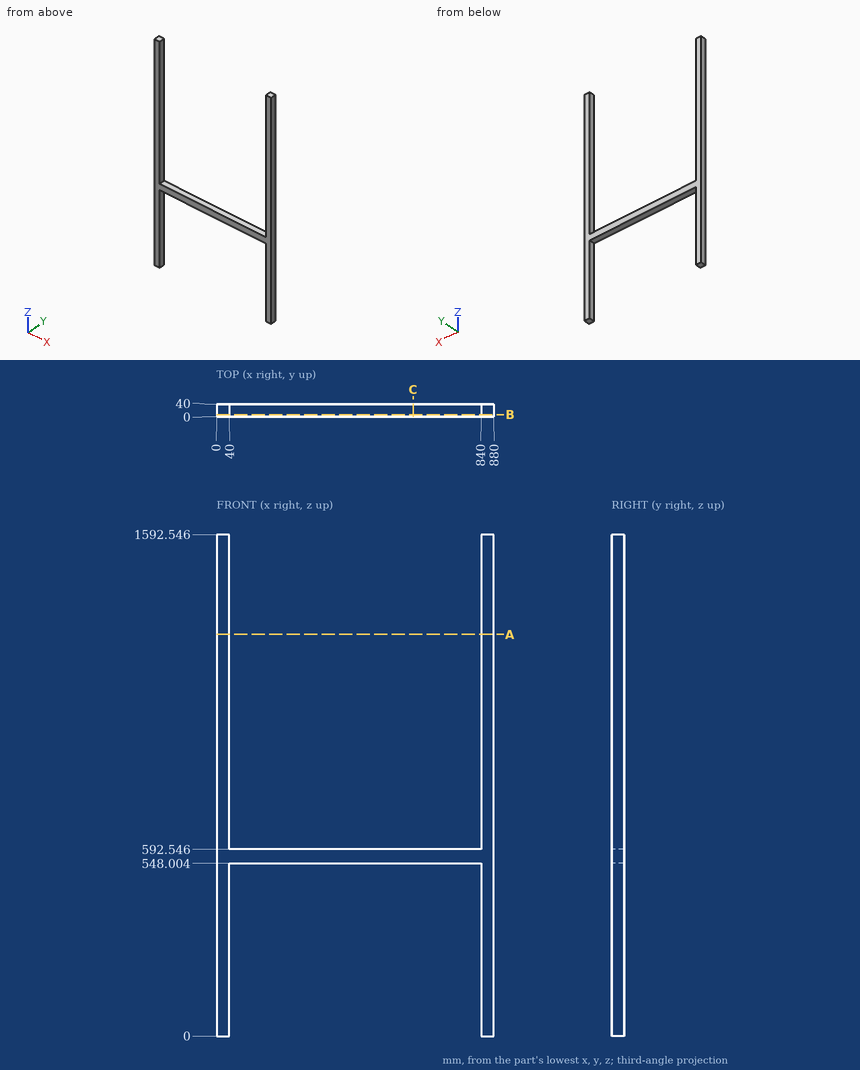
Could you check a few things on this drawing? It's one solid part, dimensions in mm from its lowest x, y, z. Give positions to 0.01 mm unless a question says otherwise; leave off trailing zeros. Write each loop counter-clockwise with the first axis right and the second up, starting at its lowest first coordinate (ties: lowest second). Pieces come first, ordered by that corner, then holes. Notation, with made-up numbers: (5.25, 29.25) -> (55.25, 29.25) arc R33 ccw to (55.25, 65.25) -> close; hole circle Ø6 at (-27.75, 86.25). An arc over 180 degrees is marked (long way). Answer as a JSON object with one key per item and string values.
Q1. Please list where these lines run through material, in increasing order: L1, parallel to X at y = 7.5, z = 769; L2, parallel to Z at x = 351.5, y = 35.
Taken from the geometry:
{"L1": "x = 0 to 40, 840 to 880", "L2": "z = 548 to 592.55"}
Q2. Suppose I cut it at C-C on x = 624. Write out the boundary of the cut face in (y, z).
Taken from the geometry:
{"outline": "(0, 548) -> (40, 548) -> (40, 592.55) -> (0, 592.55) -> close"}
Q3. Suppose I cut it at B-B on y = 6. Write out the boundary of the cut face in (x, z).
Taken from the geometry:
{"outline": "(0, 0) -> (40, 0) -> (40, 548) -> (840, 548) -> (840, 0) -> (880, 0) -> (880, 1592.55) -> (840, 1592.55) -> (840, 592.55) -> (40, 592.55) -> (40, 1592.55) -> (0, 1592.55) -> close"}
Q4. Will these pins go through, and if not, where does the flat tip stop? pin 1 Ø4 at (x, y) = (251.5, 29.5) entering from -Z; pin 2 Ø1 at (x, y) = (167, 4) entering from +Z; pin 3 Ø12 at (x, z) = (745.5, 600) entering from +Y.
Taken from the geometry:
{"pin 1": "stops at z = 548", "pin 2": "stops at z = 592.55", "pin 3": "passes through"}
Q5. Suppose I cut it at A-A on z = 1275.5. Write out the boundary of the cut face in (x, y).
Taken from the geometry:
{"outline": "(0, 0) -> (40, 0) -> (40, 40) -> (0, 40) -> close; (840, 0) -> (880, 0) -> (880, 40) -> (840, 40) -> close"}
